Verification items for the finished model (mm, model axes). Round coordinates to 2 decimals unless told otherwise and drop trailing zeros. Loops run counter-clockwise (first coordinate to the right, second up) from the corner with the lowest first, then second, coordinate; pieces in that order, holes last. Notation, with made-up numbers: (36.25, 23) - (57.25, 23) arc R35 cw to (57.25, 55) - close; hole circle Ø4 at (86.5, 23). An arc over 180 degrees is marked (long way). Use CSV: the item, a comma, the result in double quotes.
```python
from build123d import *

# Parameters (mm, degrees)
F1_DEPTH = 8
F3_R     = 11.99999
F4_D     = 5
F5_W     = 1
F5_H     = 16
F6_DEPTH = 1


# Not quite as in the source:
# - a fillet or chamfer is up to 0.001 mm smaller than in the source, because OpenCascade refuses the exact size


with BuildPart() as f1:
    # F0 (on Front) → F1 (new body, symmetric)
    with BuildSketch(Plane.XZ):
        with BuildLine():
            Line((-38.25, -6), (-33.25, -6))
            ThreePointArc((-33.25, -6), (-26.25, 1), (-19.25, -6))
            Line((-19.25, -6), (-5.2495154966, -6))
            ThreePointArc((-5.2495154966, -6), (10.875, 4), (26.9995154966, -6))
            Line((26.9995154966, -6), (41, -6))
            ThreePointArc((41, -6), (48, 1), (55, -6))
            Line((55, -6), (60, -6))
            Line((60, -6), (60, 6))
            Line((60, 6), (-38.25, 6))
            Line((-38.25, 6), (-38.25, -6))
        make_face()
    extrude(amount=F1_DEPTH, both=True)

    # F3 (radius 12 in the source; OpenCascade refuses exactly that, so slightly less here)
    f3_edges = [f1.edges().sort_by_distance(p)[0] for p in [
        (-38.25, 0, 6),
        (60, 0, 6),
    ]]
    fillet(f3_edges, radius=F3_R)

    # F4 (through all)
    with Locations(Plane.XY.offset(6)):
        with Locations((-12.25, 0), (34, 0)):
            Hole(F4_D / 2)

    # F5 (on face) → F6 (cut)
    with BuildSketch(Plane(origin=(0, 0, -6), x_dir=(1, 0, 0), z_dir=(0, 0, -1))):
        with Locations((-35.75, 0)):
            Rectangle(F5_W, F5_H)
        with Locations((57.5, 0)):
            Rectangle(F5_W, F5_H)
    extrude(amount=-F6_DEPTH, mode=Mode.SUBTRACT)


solid = f1.part
```
1) Gauge pin test, flat ends, axial feed: pin 1 Ø0.8 at (x, y) = (57.5, 1) entering from -Z; pin 2 Ø0.5 at (y, z) = (-0.5, -5.5) entering from +X; pin 3 Ø1.5 at (y, z) = (-6, 3) entering from +X. Record the tip position at first contact, or that the pin passes through.
Returned:
pin 1,"stops at z = -5"
pin 2,"stops at x = 60"
pin 3,"stops at x = 56.71"
2) Cross-section at A-A, the plane y = 0. Count the separate pieces of the cut face and the enclosed holes in it, then the cut area to 3 significant figures.
Returned:
separate pieces,"3"
enclosed holes,"0"
area,"611 mm²"
3) Cross-section at B-B, the plane x = -12.25. Record the cut outline in (y, z).
Returned:
outline,"(-8, -6) - (-2.5, -6) - (-2.5, 6) - (-8, 6) - close; (2.5, -6) - (8, -6) - (8, 6) - (2.5, 6) - close"
4) Thickness scan on probe 1 along Y at (x, z) = (-12.25, -1); probe 2 along X at (y, z) = (-0.25, 1.25); probe 3 along X at (y, z) = (-7, -4.5). Record the ranges inside material, lowest first. Write a range as [from, to].
Returned:
probe 1,"y = [-8, -2.5], [2.5, 8]"
probe 2,"x = [-35.81, -14.74], [-9.76, 1.31], [20.44, 31.51], [36.49, 57.56]"
probe 3,"x = [-38.16, -33.09], [-19.41, -4.41], [26.16, 41.16], [54.84, 59.91]"
5) Cross-section at D-D, the plane z = -0.5. Record the cut outline in (x, y), then the cut area to 3 significant figures.
Returned:
outline,"(-36.92, -8) - (-30.58, -8) - (-30.58, 8) - (-36.92, 8) - close; (-21.92, -8) - (-1.03, -8) - (-1.03, 8) - (-21.92, 8) - close; (22.78, -8) - (43.67, -8) - (43.67, 8) - (22.78, 8) - close; (52.33, -8) - (58.67, -8) - (58.67, 8) - (52.33, 8) - close; hole circle Ø5 at (-12.25, 0); hole circle Ø5 at (34, 0)"
area,"832 mm²"
6) Mould release check, pull along X, two halves, no side actions. Record for faces 1 (the face through (31.69, -0.96, -0.08)), 2 (the face through (-34.83, 0.11, 2.39)), 3 (the face through (56, 0, -6)): +X half, -X half, draft (parallel to the pull), parting line (faces both ways), or undercut.
Returned:
face 1,"undercut"
face 2,"-X half"
face 3,"draft"
